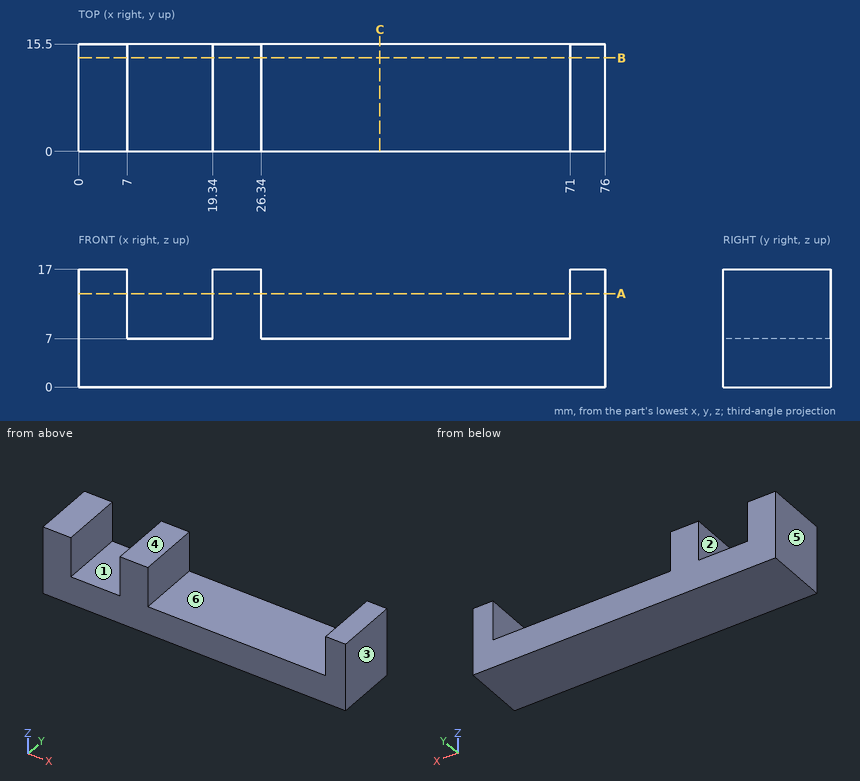
The figure shows three views and two pictorial views of one solid part (mm, origin at its lowest corner). Answer the questions. A direction names the side the tool comes from. Coordinates: 2 decimals unless noted, no trailing zeros. Loops run counter-clockwise (first coordinate to the right, second up) from the corner with the lowest first, then second, coordinate; pieces in that order, holes last. Notation, with made-up numbers: (-14, 72) -> (4, 72) arc R25 cw to (4, 100) -> close; hole circle Ø11 at (10, 89.25). An arc over 180 degrees is marked (long way). Return JSON: item names as keys, results as strings. Group by question number.
(1) A cutting plane is placed at A-A on z = 13.5. Write down the section's boundary in (x, y).
(2) A cutting plane is placed at C-C on x = 43.5. Write down the section's boundary in (y, z), and give its area (4 significant figures).
(3) Find the intervals of material crossed by probe 1 along X at (y, z) = (2.75, 10.5); probe 2 along Z at (x, y) = (63.5, 8), in increasing order. Write a range as from..to.
(4) Given pin 1 Ø2 at (x, y) = (36, 3) entering from +Z; pin 2 Ø8 at (y, z) = (7.5, 11.5) entering from -X, each flat-ended and moving along its own axis, determine where each tip first touches the part or whether it passes through.
(5) Which of the six approach directions +Z, -Z, +X, -X, +Y, -Y give full straight-line access (tool end or side, diameter ignored) to the marked faces 5 and 6?
(6) A cutting plane is placed at B-B on y = 13.5. Write down the section's boundary in (x, z), and give its area (3 significant figures).
(7) Determine the mould class of the marked faces 1, 2, 3 and 4 for opening direction X: released by +X, released by -X, zero draft, split by the parting line, or undercut.
The answers:
{
 "1": {"outline": "(0, 0) -> (7, 0) -> (7, 15.5) -> (0, 15.5) -> close; (19.34, 0) -> (26.34, 0) -> (26.34, 15.5) -> (19.34, 15.5) -> close; (71, 0) -> (76, 0) -> (76, 15.5) -> (71, 15.5) -> close"},
 "2": {"outline": "(0, 0) -> (15.5, 0) -> (15.5, 7) -> (0, 7) -> close", "area": "108.5 mm^2"},
 "3": {"probe 1": "x = 0..7, 19.34..26.34, 71..76", "probe 2": "z = 0..7"},
 "4": {"pin 1": "stops at z = 7", "pin 2": "stops at x = 0"},
 "5": {"face 5": "+Z, -Z, -X, +Y, -Y", "face 6": "+Z, +Y, -Y"},
 "6": {"outline": "(0, 0) -> (76, 0) -> (76, 17) -> (71, 17) -> (71, 7) -> (26.34, 7) -> (26.34, 17) -> (19.34, 17) -> (19.34, 7) -> (7, 7) -> (7, 17) -> (0, 17) -> close", "area": "722 mm^2"},
 "7": {"face 1": "undercut", "face 2": "undercut", "face 3": "released by +X", "face 4": "zero draft"}
}
